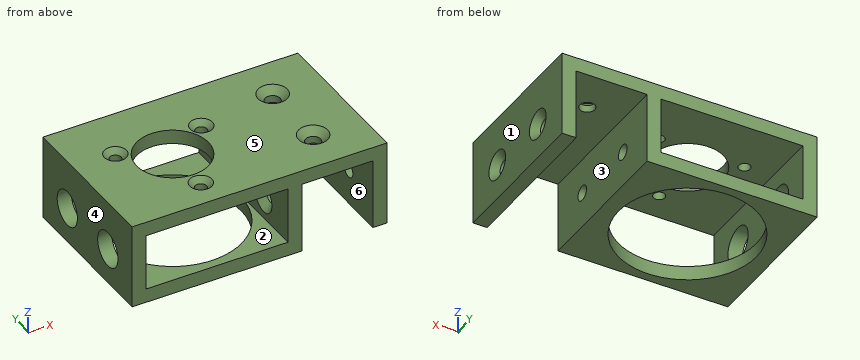
from build123d import *

# Parameters (mm, degrees)
SKETCH1_W           = 40
SKETCH1_H           = 16
BOSS_EXTRUDE1_DEPTH = 44
CUT_EXTRUDE1_REACH  = 86.475
SKETCH3_R           = 19.5
CUT_EXTRUDE2_REACH  = 86.475
SKETCH4_R           = 10.15
SKETCH4_R_2         = 1.625
SKETCH5_R           = 2.125
CUT_EXTRUDE3_DEPTH  = 87.717933555
CUT_EXTRUDE4_REACH  = 86.475
SKETCH6_R           = 2.125
CHAMFER1_SIZE       = 2
CHAMFER2_SIZE       = 1.5
CUT_EXTRUDE5_REACH  = 88.718
SKETCH7_R           = 5


with BuildPart() as part:
    # Sketch1 → Boss-Extrude1 (new body)
    with BuildSketch(Plane(origin=(0, 0, 0), x_dir=(1, 0, 0), z_dir=(0, 1, 0))):
        Polygon((0, 0), (0, 20), (4, 20), (4, -4), (-24, -4), (-68, -4), (-68, 0), (-68, 16), (-68, 20), (-24, 20), (-20, 20), (-20, 0), align=None)
        with Locations((-44, 8)):
            Rectangle(SKETCH1_W, SKETCH1_H, mode=Mode.SUBTRACT)
    extrude(amount=BOSS_EXTRUDE1_DEPTH)

    # Sketch3 → Cut-Extrude1 (cut, up to next)
    with BuildSketch(Plane(origin=(0, 0, -20), x_dir=(-1, 0, 0), z_dir=(0, 0, -1)), mode=Mode.PRIVATE) as cut_extrude1_sk1:
        with Locations((44, 22)):
            Circle(SKETCH3_R)
    cut_extrude1_tool1 = extrude(cut_extrude1_sk1.sketch, amount=-CUT_EXTRUDE1_REACH, mode=Mode.PRIVATE) & part.part
    add(cut_extrude1_tool1.solids().sort_by_distance((-44, 22, -20))[0], mode=Mode.SUBTRACT)

    # Sketch4 → Cut-Extrude2 (cut, up to next)
    with BuildSketch(Plane.XY.offset(4), mode=Mode.PRIVATE) as cut_extrude2_sk1:
        with Locations((-44, 22)):
            Circle(SKETCH4_R)
    cut_extrude2_tool1 = extrude(cut_extrude2_sk1.sketch, amount=-CUT_EXTRUDE2_REACH, mode=Mode.PRIVATE) & part.part
    # Sketch4 → Cut-Extrude2 (cut, up to next)
    with BuildSketch(Plane.XY.offset(4), mode=Mode.PRIVATE) as cut_extrude2_sk2:
        with Locations((-56.124355653, 29)):
            Circle(SKETCH4_R_2)
    cut_extrude2_tool2 = extrude(cut_extrude2_sk2.sketch, amount=-CUT_EXTRUDE2_REACH, mode=Mode.PRIVATE) & part.part
    # Sketch4 → Cut-Extrude2 (cut, up to next)
    with BuildSketch(Plane.XY.offset(4), mode=Mode.PRIVATE) as cut_extrude2_sk3:
        with Locations((-31.875644347, 29)):
            Circle(SKETCH4_R_2)
    cut_extrude2_tool3 = extrude(cut_extrude2_sk3.sketch, amount=-CUT_EXTRUDE2_REACH, mode=Mode.PRIVATE) & part.part
    # Sketch4 → Cut-Extrude2 (cut, up to next)
    with BuildSketch(Plane.XY.offset(4), mode=Mode.PRIVATE) as cut_extrude2_sk4:
        with Locations((-44, 8)):
            Circle(SKETCH4_R_2)
    cut_extrude2_tool4 = extrude(cut_extrude2_sk4.sketch, amount=-CUT_EXTRUDE2_REACH, mode=Mode.PRIVATE) & part.part
    add(cut_extrude2_tool1.solids().sort_by_distance((-44, 22, 4))[0], mode=Mode.SUBTRACT)
    add(cut_extrude2_tool2.solids().sort_by_distance((-56.124356, 29, 4))[0], mode=Mode.SUBTRACT)
    add(cut_extrude2_tool3.solids().sort_by_distance((-31.875644, 29, 4))[0], mode=Mode.SUBTRACT)
    add(cut_extrude2_tool4.solids().sort_by_distance((-44, 8, 4))[0], mode=Mode.SUBTRACT)

    # Sketch5 → Cut-Extrude3 (cut, through all)
    with BuildSketch(Plane(origin=(4, 0, 0), x_dir=(0, 0, -1), z_dir=(1, 0, 0))):
        with Locations(Location((10, 32, 0), (0, 0, 180))):
            Circle(SKETCH5_R)
        with Locations(Location((10, 12, 0), (0, 0, 180))):
            Circle(SKETCH5_R)
    extrude(amount=-CUT_EXTRUDE3_DEPTH, mode=Mode.SUBTRACT)

    # Sketch6 → Cut-Extrude4 (cut, up to next)
    with BuildSketch(Plane.XY.offset(4), mode=Mode.PRIVATE) as cut_extrude4_sk1:
        with Locations((-10, 32)):
            Circle(SKETCH6_R)
    cut_extrude4_tool1 = extrude(cut_extrude4_sk1.sketch, amount=-CUT_EXTRUDE4_REACH, mode=Mode.PRIVATE) & part.part
    # Sketch6 → Cut-Extrude4 (cut, up to next)
    with BuildSketch(Plane.XY.offset(4), mode=Mode.PRIVATE) as cut_extrude4_sk2:
        with Locations((-10, 12)):
            Circle(SKETCH6_R)
    cut_extrude4_tool2 = extrude(cut_extrude4_sk2.sketch, amount=-CUT_EXTRUDE4_REACH, mode=Mode.PRIVATE) & part.part
    add(cut_extrude4_tool1.solids().sort_by_distance((-10, 32, 4))[0], mode=Mode.SUBTRACT)
    add(cut_extrude4_tool2.solids().sort_by_distance((-10, 12, 4))[0], mode=Mode.SUBTRACT)

    # Chamfer1
    chamfer1_edges = [part.edges().sort_by_distance(p)[0] for p in [
        (-12.125, 12, 4),
        (-24, 32, -12.125),
        (4, 32, -12.125),
        (-24, 12, -12.125),
        (4, 12, -12.125),
        (-12.125, 32, 4),
    ]]
    chamfer(chamfer1_edges, length=CHAMFER1_SIZE)

    # Chamfer2
    chamfer2_edges = [part.edges().sort_by_distance(p)[0] for p in [
        (-45.625, 8, 4),
        (-33.500644347, 29, 4),
        (-57.749355653, 29, 4),
    ]]
    chamfer(chamfer2_edges, length=CHAMFER2_SIZE)

    # Sketch7 → Cut-Extrude5 (cut, up to next)
    with BuildSketch(Plane.ZY.offset(68), mode=Mode.PRIVATE) as cut_extrude5_sk1:
        with Locations((-10, 32)):
            Circle(SKETCH7_R)
    cut_extrude5_tool1 = extrude(cut_extrude5_sk1.sketch, amount=-CUT_EXTRUDE5_REACH, mode=Mode.PRIVATE) & part.part
    # Sketch7 → Cut-Extrude5 (cut, up to next)
    with BuildSketch(Plane.ZY.offset(68), mode=Mode.PRIVATE) as cut_extrude5_sk2:
        with Locations((-10, 12)):
            Circle(SKETCH7_R)
    cut_extrude5_tool2 = extrude(cut_extrude5_sk2.sketch, amount=-CUT_EXTRUDE5_REACH, mode=Mode.PRIVATE) & part.part
    add(cut_extrude5_tool1.solids().sort_by_distance((-68, 32, -10))[0], mode=Mode.SUBTRACT)
    add(cut_extrude5_tool2.solids().sort_by_distance((-68, 12, -10))[0], mode=Mode.SUBTRACT)


solid = part.part
Input: part model. Units: mm. Frame: model coordinates. Face numbers are marked on the shaded views. A direction names the side the tool comes from. Coordinates: 2 decimals unless noted, no trailing zeros. Loops run counter-clockwise (first coordinate to the right, second up) from the corner with the lowest first, then second, coordinate; pieces in that order, holes last. Notation, with made-up numbers: (86, 4) -> (121, 4) arc R25 ccw to (121, 26) -> close; hole circle Ø2 at (41.25, 82.5). An arc over 180 degrees is marked (long way). Write each question's results on one line, items separated by ' | '. Start each with the question number.
Q1. Reachability of the marked faces 1, 2 and 3 from +Z, -Z, +X, -X, +Y, -Y: full face, straight path, thin tool, end or side. Return the list, or none.
Q2. Section A-A, the plane z = -1.75. Return the cut outline in (x, y).
Q3. Section B-B, the plane x = -10. Return the cut outline in (y, z) (3 decimals), plus the area to 3 significant figures.
Q4. Pin query (flat end, axial travel): pin 1 (3.5 mm diameter, centred on x = -44, y = 8, fed in from +Z) (3 decimals); pin 2 (2.5 mm diameter, centred on y = 12, z = -10, fed in from -X); pin 3 (5 mm diameter, centred on x = -56.12, y = 29, fed in from -Z); pin 4 (8 mm diameter, centred on x = -33.5, y = 28.5, fed in from +Z). Return the tip coordinate at first contact, or that it passes through.
Q5. Section D-D, the plane x = -44. Return the cut outline in (y, z) (3 decimals).
Q6. Section C-C, the plane z = -18. Return the cut outline in (x, y).
Q7. Pull-direction query (X, two-part tool) for the marked faces 4, 5 and 6; classes: released by +X, released by -X, zero draft, split by the parting line, or undercut.
Q8. Ray query, line 1 (X direction, y = 7, z = -5.25); line 2 (Y direction, x = -10, z = 1.25) (3 decimals); line 3 (Z direction, x = 1.15, y = 12) (3 decimals). Return the intervals inside material, ascending. Write a range as from..to.
Found:
1) face 1: +Z, -Z, +X, +Y, -Y | face 2: +Y, -Y | face 3: -Z, +Y, -Y
2) outline: (-68, 0) -> (-64, 0) -> (-64, 44) -> (-68, 44) -> close; (-24, 0) -> (-20, 0) -> (-20, 44) -> (-24, 44) -> close; (0, 0) -> (4, 0) -> (4, 44) -> (0, 44) -> close
3) outline: (0, 0) -> (9.875, 0) -> (9.875, 2) -> (7.875, 4) -> (0, 4) -> close; (14.125, 0) -> (29.875, 0) -> (29.875, 2) -> (27.875, 4) -> (16.125, 4) -> (14.125, 2) -> close; (34.125, 0) -> (44, 0) -> (44, 4) -> (36.125, 4) -> (34.125, 2) -> close | area: 134 mm2
4) pin 1: z = 2.625 | pin 2: through | pin 3: z = 0 | pin 4: z = 4
5) outline: (0, -20) -> (2.5, -20) -> (2.5, -16) -> (0, -16) -> close; (0, 0) -> (6.375, 0) -> (6.375, 2.5) -> (4.875, 4) -> (0, 4) -> close; (9.625, 0) -> (11.85, 0) -> (11.85, 4) -> (11.125, 4) -> (9.625, 2.5) -> close; (32.15, 0) -> (44, 0) -> (44, 4) -> (32.15, 4) -> close; (41.5, -20) -> (44, -20) -> (44, -16) -> (41.5, -16) -> close
6) outline: (-68, 0) -> (-20, 0) -> (-20, 44) -> (-68, 44) -> close; (0, 0) -> (4, 0) -> (4, 44) -> (0, 44) -> close; hole circle Ø39 at (-44, 22)
7) face 4: released by -X | face 5: zero draft | face 6: undercut
8) line 1: -68..-64, -24..-20, 0..4 | line 2: 0..9.875, 14.125..29.875, 34.125..44 | line 3: -20..-12.125, -7.875..4
